The model under review builds one solid part; all positions refer to its coordinate system, in mm. Face numbers are marked on the shaded views. A direction names the side the tool comes from. Round coordinates to 2 decimals unless told otherwise and drop trailing zeros. Loops run counter-clockwise (first coordinate to the right, second up) from the corner with the lowest first, then second, coordinate; pieces in that order, holes last. Notation, with made-up numbers: (9, 67) -> (42, 67) arc R29 ccw to (42, 96) -> close; hole circle Ø5 at (-28.75, 72). An arc over 180 degrees is marked (long way). Write each question's results on one line, items separated by ' | '. Start each with the question number.
Item 1: Mouldability with a two-part tool opening along Y and no side actions: class the marked faces 1, 2 and 3 as pulls with the +Y half, pulls with the -Y half, needs draft (parallel to the pull), parting line crosses it, or undercut.
Item 2: Clearance check with flat-ended pins moving along their axes: pin 1 Ø5 at (x, y) = (4.5, 28) entering from -Z; pin 2 Ø2 at (y, z) = (4, 54) entering from +X; pin 3 Ø12 at (x, z) = (26.5, 10) entering from +Y. State where each tip first meets the part, or that it passes through.
Item 3: Tool access review of the marked faces 4 and 5: name each direction out of +Z, -Z, +X, -X, +Y, -Y from which nothing blocks a thin tool from reaching the whole face with its end or side.
Item 4: For L1, parallel to Z at x = -35, y = 31; L2, parallel to Z at x = 26.5, y = 12; L3, parallel to X at y = 10.5, z = -30.5, list the stretches that pass through material, from the lowest coordinate up. Write a range as from..to.
Item 5: We need section D-D (z = 39). Give the boundary of the cut face in (x, y), and give its area (3 significant figures).
Item 6: We need section C-C (x = 11.5). Give the boundary of the cut face in (y, z).
Item 7: We need section A-A (x = 0). Give the boundary of the cut face in (y, z).
Item 8: We need section B-B (z = -44.75). Give the boundary of the cut face in (x, y).
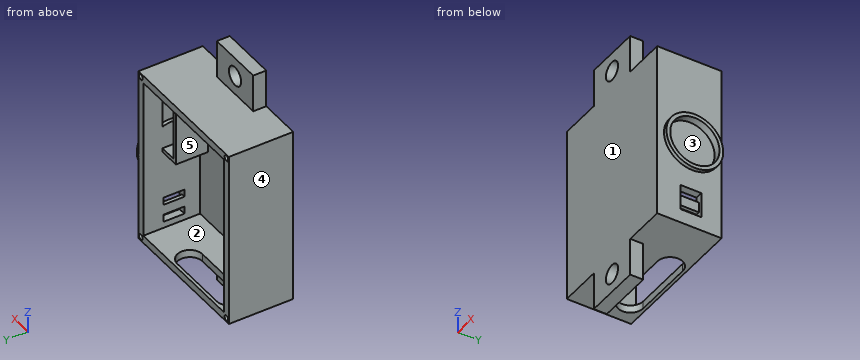
from build123d import *

# Parameters (mm, degrees)
SKETCH2_W           = 74.5
SKETCH2_H           = 93.5
BOSS_EXTRUDE1_DEPTH = 34
SHELL1_T            = -4
SKETCH4_R           = 15
BOSS_EXTRUDE2_DEPTH = 2
SHELL2_START        = 35.25
SHELL2_OUTLINE_R    = 13
SHELL2_DEPTH        = 4
SKETCH5_W           = 33
SKETCH5_H           = 17
BOSS_EXTRUDE3_DEPTH = 11
SHELL3_START        = 24.25
SHELL3_OUTLINE_W    = 15
SHELL3_OUTLINE_H    = 29
SHELL3_DEPTH        = 9
SHELL3_START_2      = 33.25
SHELL3_2_DEPTH      = 2
SKETCH8_W           = 4.5
SKETCH8_H           = 15
CUT_EXTRUDE1_DEPTH  = 7
SKETCH9_R           = 1.5
CUT_EXTRUDE3_DEPTH  = 7
SKETCH10_W          = 13.5
SKETCH10_H          = 11
CUT_EXTRUDE5_DEPTH  = 2
SKETCH11_W          = 4
SKETCH11_H          = 11
CUT_EXTRUDE6_DEPTH  = 12
CUT_EXTRUDE7_DEPTH  = 10
SKETCH13_W          = 30
SKETCH13_H          = 6.856904394
BOSS_EXTRUDE6_DEPTH = 20
SKETCH19_W          = 30
SKETCH19_H          = 6.86
BOSS_EXTRUDE7_DEPTH = 20
SKETCH20_R          = 5
CUT_EXTRUDE8_DEPTH  = 20
SKETCH21_R          = 5
CUT_EXTRUDE9_DEPTH  = 20


# Read off the part's stored shape, not the designer's step: Shell2, Shell3
with BuildPart() as part:
    # Sketch2 → Boss-Extrude1 (new body)
    with BuildSketch(Plane(origin=(0, 0, 0), x_dir=(1, 0, 0), z_dir=(0, 1, 0))):
        Rectangle(SKETCH2_W, SKETCH2_H)
    extrude(amount=BOSS_EXTRUDE1_DEPTH)

    # Shell1
    shell1_openings = [part.faces().sort_by_distance(p)[0] for p in [
        (0, 34, 0),
    ]]
    offset(amount=SHELL1_T, openings=shell1_openings, kind=Kind.INTERSECTION)

    # Sketch4 → Boss-Extrude2 (add)
    with BuildSketch(Plane(origin=(37.25, 0, 0), x_dir=(0, 0, -1), z_dir=(1, 0, 0))):
        with Locations((0, 18.6)):
            Circle(SKETCH4_R)
    extrude(amount=BOSS_EXTRUDE2_DEPTH)

    # Shell2 outline → Shell2 (cut)
    with BuildSketch(Plane.YZ.offset(SHELL2_START)):
        with Locations((18.6, 0)):
            Circle(SHELL2_OUTLINE_R)
    extrude(amount=SHELL2_DEPTH, mode=Mode.SUBTRACT)

    # Sketch5 → Boss-Extrude3 (add)
    with BuildSketch(Plane.ZY.offset(-33.25)):
        with Locations((16.5, 15.356904394)):
            Rectangle(SKETCH5_W, SKETCH5_H)
    extrude(amount=BOSS_EXTRUDE3_DEPTH)

    # Shell3 outline → Shell3 (cut)
    with BuildSketch(Plane.YZ.offset(SHELL3_START)):
        with Locations((16.356904394, 16.5)):
            Rectangle(SHELL3_OUTLINE_W, SHELL3_OUTLINE_H)
    extrude(amount=SHELL3_DEPTH, mode=Mode.SUBTRACT)

    # Shell3 2 outline → Shell3 2 (cut)
    with BuildSketch(Plane.YZ.offset(SHELL3_START_2)):
        with BuildLine():
            Line((8.856904394, 31), (8.856904394, 11.404915081))
            ThreePointArc((8.856904394, 11.404915081), (15.996381403, 14.77231093), (23.856904394, 14.048663858))
            Line((23.856904394, 14.048663858), (23.856904394, 31))
            Line((23.856904394, 31), (8.856904394, 31))
        make_face()
    extrude(amount=SHELL3_2_DEPTH, mode=Mode.SUBTRACT)

    # Sketch8 → Cut-Extrude1 (cut)
    with BuildSketch(Plane(origin=(0, 0, 31), x_dir=(-1, 0, 0), z_dir=(0, 0, -1))):
        with Locations((-26.5, 16.356904394)):
            Rectangle(SKETCH8_W, SKETCH8_H)
    extrude(amount=-CUT_EXTRUDE1_DEPTH, mode=Mode.SUBTRACT)

    # Sketch9 → Cut-Extrude3 (cut)
    with BuildSketch(Plane(origin=(0, 34, 0), x_dir=(1, 0, 0), z_dir=(0, 1, 0))):
        with Locations(Location((-35.25, -44.75, 0), (0, 0, 270))):
            Circle(SKETCH9_R)
        with Locations(Location((35.25, -44.75, 0), (0, 0, 270))):
            Circle(SKETCH9_R)
        with Locations(Location((35.25, 44.75, 0), (0, 0, 270))):
            Circle(SKETCH9_R)
        with Locations(Location((-35.25, 44.75, 0), (0, 0, 270))):
            Circle(SKETCH9_R)
    extrude(amount=-CUT_EXTRUDE3_DEPTH, mode=Mode.SUBTRACT)

    # Sketch10 → Cut-Extrude5 (cut)
    with BuildSketch(Plane(origin=(37.25, 0, 0), x_dir=(0, 0, -1), z_dir=(1, 0, 0))):
        with Locations((32.604466308, 17.811561776)):
            Rectangle(SKETCH10_W, SKETCH10_H)
    extrude(amount=-CUT_EXTRUDE5_DEPTH, mode=Mode.SUBTRACT)

    # Sketch11 → Cut-Extrude6 (cut)
    with BuildSketch(Plane(origin=(35.25, 0, 0), x_dir=(0, 0, -1), z_dir=(1, 0, 0))):
        with Locations((27.854466308, 17.811561776)):
            Rectangle(SKETCH11_W, SKETCH11_H)
        with Locations((37.354466308, 17.811561776)):
            Rectangle(SKETCH11_W, SKETCH11_H)
    extrude(amount=-CUT_EXTRUDE6_DEPTH, mode=Mode.SUBTRACT)

    # Sketch12 → Cut-Extrude7 (cut)
    with BuildSketch(Plane(origin=(0, 0, -46.75), x_dir=(-1, 0, 0), z_dir=(0, 0, -1))):
        with BuildLine():
            Line((-7.742051662, 32.367861053), (24.842051662, 32.367861053))
            ThreePointArc((24.842051662, 32.367861053), (31.467861053, 25.742051662), (24.842051662, 19.11624227))
            Line((24.842051662, 19.11624227), (-7.742051662, 19.11624227))
            ThreePointArc((-7.742051662, 19.11624227), (-14.367861053, 25.742051662), (-7.742051662, 32.367861053))
        make_face()
    extrude(amount=-CUT_EXTRUDE7_DEPTH, mode=Mode.SUBTRACT)

    # Sketch13 → Boss-Extrude6 (add)
    with BuildSketch(Plane(origin=(0, 0, -46.75), x_dir=(-1, 0, 0), z_dir=(0, 0, -1))):
        with Locations((0, 3.428452197)):
            Rectangle(SKETCH13_W, SKETCH13_H)
    extrude(amount=BOSS_EXTRUDE6_DEPTH)

    # Sketch19 → Boss-Extrude7 (add)
    with BuildSketch(Plane.XY.offset(46.75)):
        with Locations((0, 3.43)):
            Rectangle(SKETCH19_W, SKETCH19_H)
    extrude(amount=BOSS_EXTRUDE7_DEPTH)

    # Sketch20 → Cut-Extrude8 (cut)
    with BuildSketch(Plane(origin=(0, 6.856904394, 0), x_dir=(1, 0, 0), z_dir=(0, 1, 0))):
        with Locations(Location((0, 56.75, 0), (0, 0, 270))):
            Circle(SKETCH20_R)
    extrude(amount=-CUT_EXTRUDE8_DEPTH, mode=Mode.SUBTRACT)

    # Sketch21 → Cut-Extrude9 (cut)
    with BuildSketch(Plane(origin=(0, 6.86, 0), x_dir=(1, 0, 0), z_dir=(0, 1, 0))):
        with Locations(Location((0, -56.75, 0), (0, 0, 270))):
            Circle(SKETCH21_R)
    extrude(amount=-CUT_EXTRUDE9_DEPTH, mode=Mode.SUBTRACT)


solid = part.part
Here are the results:
1) face 1: pulls with the -Y half | face 2: needs draft | face 3: undercut
2) pin 1: stops at z = 42.75 | pin 2: stops at x = 15 | pin 3: stops at y = 23.86
3) face 4: +Z, -Z, -X, +Y, -Y | face 5: +Y
4) L1: z = -46.75..-46.23, -43.27..43.27, 46.23..46.75 | L2: z = -46.75..-42.75, 0..2, 42.75..46.75 | L3: x = -37.25..-33.25, 33.25..37.25
5) outline: (-37.25, 0) -> (37.25, 0) -> (37.25, 34) -> (33.25, 34) -> (33.25, 4) -> (-33.25, 4) -> (-33.25, 34) -> (-37.25, 34) -> close | area: 538 mm2
6) outline: (0, -66.75) -> (6.86, -66.75) -> (6.86, -46.75) -> (20.29, -46.75) -> (20.29, -42.75) -> (4, -42.75) -> (4, 42.75) -> (34, 42.75) -> (34, 46.75) -> (6.86, 46.75) -> (6.86, 66.75) -> (0, 66.75) -> close; (31.2, -46.75) -> (34, -46.75) -> (34, -42.75) -> (31.2, -42.75) -> close
7) outline: (0, -66.75) -> (6.86, -66.75) -> (6.86, -61.75) -> (0, -61.75) -> close; (0, -51.75) -> (6.86, -51.75) -> (6.86, -46.75) -> (19.12, -46.75) -> (19.12, -42.75) -> (4, -42.75) -> (4, 42.75) -> (34, 42.75) -> (34, 46.75) -> (6.86, 46.75) -> (6.86, 51.75) -> (0, 51.75) -> close; (0, 61.75) -> (6.86, 61.75) -> (6.86, 66.75) -> (0, 66.75) -> close; (32.37, -46.75) -> (34, -46.75) -> (34, -42.75) -> (32.37, -42.75) -> close
8) outline: (-37.25, 0) -> (37.25, 0) -> (37.25, 34) -> (36.75, 34) -> (36.75, 27) -> (33.75, 27) -> (33.75, 34) -> (-33.75, 34) -> (-33.75, 27) -> (-36.75, 27) -> (-36.75, 34) -> (-37.25, 34) -> close; hole (-24.84, 19.12) -> (7.74, 19.12) arc R6.63 ccw to (7.74, 32.37) -> (-24.84, 32.37) arc R6.63 ccw to start
